from build123d import *

# Parameters (mm, degrees)
SKETCH1_R           = 4
BOSS_EXTRUDE1_DEPTH = 8
SKETCH2_R           = 7.5
BOSS_EXTRUDE2_DEPTH = 5
BOSS_EXTRUDE3_START = 6
SKETCH3_R           = 4
BOSS_EXTRUDE3_DEPTH = 6
SKETCH4_W           = 0.5
SKETCH4_H           = 0.7


with BuildPart() as part:
    # Sketch1 → Boss-Extrude1 (new body)
    with BuildSketch(Plane.XY):
        Circle(SKETCH1_R)
    extrude(amount=BOSS_EXTRUDE1_DEPTH)

    # Sketch2 → Boss-Extrude2 (add)
    with BuildSketch(Plane(origin=(0, 0, 0), x_dir=(-1, 0, 0), z_dir=(0, 0, -1))):
        Circle(SKETCH2_R)
    extrude(amount=BOSS_EXTRUDE2_DEPTH)

    # Sketch3 → Boss-Extrude3 (add)
    with BuildSketch(Plane(origin=(0, 0, -5), x_dir=(-1, 0, 0), z_dir=(0, 0, -1)).offset(BOSS_EXTRUDE3_START)):
        with Locations(Location((0, 0, 0), (0, 0, 180))):
            Circle(SKETCH3_R)
    extrude(amount=-BOSS_EXTRUDE3_DEPTH)

    # Sketch4 → Cut-Revolve1 (revolve, cut)
    with BuildSketch(Plane(origin=(0, 0, 0), x_dir=(1, 0, 0), z_dir=(0, 1, 0)), mode=Mode.PRIVATE) as cut_revolve1_sk:
        with Locations((-3.75, -5.75)):
            Rectangle(SKETCH4_W, SKETCH4_H)
        with Locations((-3.75, 9.25)):
            Rectangle(SKETCH4_W, SKETCH4_H)
    revolve(cut_revolve1_sk.sketch.rotate(Axis((0, 0, 0), (0, 0, -1)), 180), axis=Axis((0, 0, 0), (0, 0, -1)), mode=Mode.SUBTRACT)


solid = part.part
Geometry check sheet. Reference: the model listing, model coordinates, mm. A direction names the side the tool comes from. Give positions to 0.01 mm unless a question says otherwise; leave off trailing zeros. Write each loop counter-clockwise with the first axis right and the second up, starting at its lowest first coordinate (ties: lowest second). Pieces come first, ordered by that corner, then holes. Notation, with made-up numbers: M 64.25,-3 L 72.25,-3 A35 cw 72.25,33 Z; hole C -28,-21 d8. An arc over 180 degrees is marked long. Answer as CSV lines item,"result". Start each with the question number.
Q1. Section check A-A, the plane x = 0. Record the cut outline in (y, z), then the cut area to 3 significant figures.
Q2. Go/stop test with flat-tipped pins: pin 1 (3 mm diameter, centred on x = -1.5, z = -6, fed in from -Y); pin 2 (3 mm diameter, centred on x = -4.5, z = -6, fed in from -Y); pin 3 (4 mm diameter, centred on x = -4.5, y = 5.5, fed in from +Z); pin 4 (3 mm diameter, centred on x = 5, y = 0, fed in from +Z). Record where each tip stops, or that it passes through.
Q3. Section check C-C, the plane z = -4. Record the cut outline in (x, y).
Q4. Material ranges on L1, parallel to Z at x = -6.5, y = 0.25; L2, parallel to X at y = -3.25, z = -7.25; L3, parallel to X at y = 1.5, z = -6.75, recorded low to high.
Q5. Tool access check on faces 4 (the face through (-0.867, -3.905, 7.037)), 5 (the face through (3.233, 1.341, 5.745)), 6 (the face through (7.493, 0.33, -2.465)), 7 (the face through (-3, -3, -5)). Record the directions out of +Z, -Z, +X, -X, +Y, -Y that give a thin tool (end or side, any length) a straight path to the whole face; none if there is none.
Q6. Section check D-D, the plane y = -4.5. Record the cut outline in (x, z), then the cut area to 3 significant figures.
Q7. Release check for a two-part mould opening along Z. For faces 1 (the face through (0, 0, -11)), 2 (the face through (3.233, 1.341, -9.255)), 3 (the face through (-0.867, -3.905, 2.662)) record: pulls with the +Z half, pulls with the -Z half, needs draft (parallel to the pull), parting line crosses it, or undercut.
Geometry says:
1,outline,"M -7.5,-5 L -4,-5 L -4,-8.9 L -3.5,-8.9 L -3.5,-9.6 L -4,-9.6 L -4,-11 L 4,-11 L 4,-9.6 L 3.5,-9.6 L 3.5,-8.9 L 4,-8.9 L 4,-5 L 7.5,-5 L 7.5,0 L 4,0 L 4,5.4 L 3.5,5.4 L 3.5,6.1 L 4,6.1 L 4,8 L -4,8 L -4,6.1 L -3.5,6.1 L -3.5,5.4 L -4,5.4 L -4,0 L -7.5,0 Z"
1,area,"186 mm^2"
2,pin 1,"y = -7.49"
2,pin 2,"y = -6.69"
2,pin 3,"z = 0"
2,pin 4,"z = 8"
3,outline,"C 0,0 d15"
4,L1,"-5 to 0"
4,L2,"-2.33 to 2.33"
4,L3,"-3.71 to 3.71"
5,face 4,"+Z"
5,face 5,"none"
5,face 6,"+Z, -Z"
5,face 7,"-Z"
6,outline,"M -6,-5 L 6,-5 L 6,0 L -6,0 Z"
6,area,"60.0 mm^2"
7,face 1,"pulls with the -Z half"
7,face 2,"undercut"
7,face 3,"needs draft"
